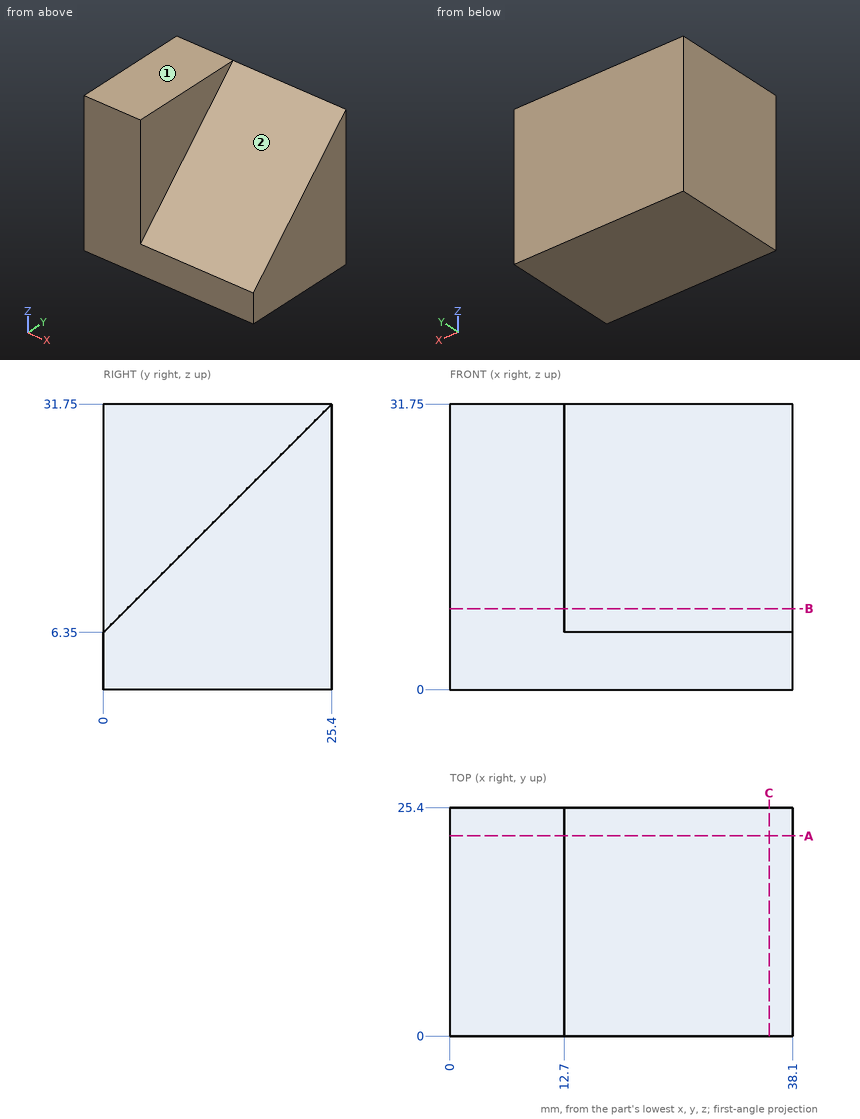
For this review, use the dimensioned drawing (mm, ordinates from the lowest corner) and the shaded views. A direction names the side the tool comes from. Coordinates: 2 decimals unless noted, no trailing zeros. Order: outer loops, then holes, each group sorted by start corner. A loop starts at its lowest first (then second) coordinate and runs counter-clockwise, first axis right, second up. Notation, with made-up numbers: (54.5, 53) - (98.5, 53) arc R33 cw to (98.5, 90) - close; hole circle Ø11 at (4.25, 17.5). An arc over 180 degrees is marked (long way). Answer in a Markdown table with one row per item.
(1) Consider section A-A on y = 22.25. State the section outline as (x, z) points, plus the area to 3 significant figures.
Checked values:
| item | result |
|---|---|
| outline | (0, 0) - (38.1, 0) - (38.1, 28.6) - (12.7, 28.6) - (12.7, 31.75) - (0, 31.75) - close |
| area | 1,130 mm^2 |
(2) Consider section C-C on x = 35.5. State the section outline as (y, z) points.
Checked values:
| item | result |
|---|---|
| outline | (0, 0) - (25.4, 0) - (25.4, 31.75) - (0, 6.35) - close |
(3) Consider section B-B on z = 9. State the section outline as (x, y) points, plus the area to 3 significant figures.
Checked values:
| item | result |
|---|---|
| outline | (0, 0) - (12.7, 0) - (12.7, 2.65) - (38.1, 2.65) - (38.1, 25.4) - (0, 25.4) - close |
| area | 900 mm^2 |
(4) For the marked faces 1 and 2, list the 3-axis set-ups (+Z, -Z, +X, -X, +Y, -Y) from which the entire face can be reached by the end or side of a thin tool; tool diameter is ignored.
Checked values:
| item | result |
|---|---|
| face 1 | +Z, +X, -X, +Y, -Y |
| face 2 | +Z, +X, -Y |
(5) Clearance check with flat-ended pins moving along their axes: pin 1 (6 mm diameter, centred on y = 7, z = 21.5, fed in from -X); pin 2 (5 mm diameter, centred on y = 10.5, z = 25, fed in from +X); pin 3 (3 mm diameter, centred on x = 29, y = 8, fed in from +Z). State where each tip first meets the part, or that it passes through.
Checked values:
| item | result |
|---|---|
| pin 1 | x = 0 |
| pin 2 | x = 12.7 |
| pin 3 | z = 15.85 |
(6) Wall thickness on line 1 along X through (y, z) = (6.5, 15.5); line 2 along Z through (x, y) = (31, 5.75); line 3 along Y through (x, z) = (33.5, 27): over which ranges is each line inside the solid? List them lowest first. Write a range as from..to.
Checked values:
| item | result |
|---|---|
| line 1 | 0..12.7 |
| line 2 | 0..12.1 |
| line 3 | 20.65..25.4 |
